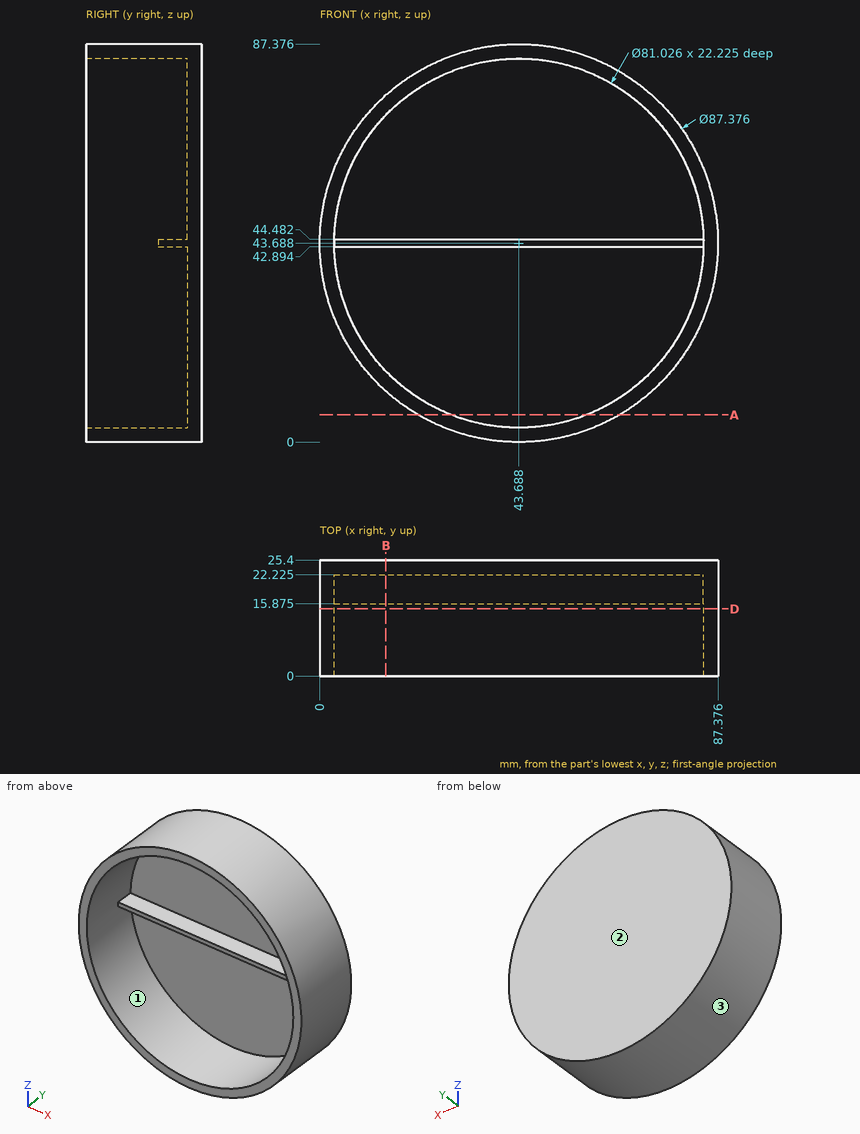
Answer from the drawing. Dimensions are ordinates in mm from the lowest x, y and z of the part. Coordinates: 2 decimals unless noted, no trailing zeros. Order: outer loops, then holes, each group sorted by start corner. A loop starts at its lowest first (then second) coordinate and runs counter-clockwise, first axis right, second up. Notation, with made-up numbers: (-38.5, 83) - (17.5, 83) arc R30 cw to (17.5, 117) - close; hole circle Ø9 at (38.25, 21). An arc over 180 degrees is marked (long way). Answer as a JSON object with one key per item and string values. Group by question number.
Item 1: Consider probe 1 along Z at (x, y) = (43.5, 4.5) (1 decimal); probe 2 along Y at (x, z) = (31.5, 46.5) (1 decimal); probe 3 along X at (y, z) = (18.25, 16) (1 decimal). Determine where each line is inside the solid, lowest interval first. Write a range as from..to.
Item 2: Section A-A (z = 6) is taken. Give the vertices of the cut face in (x, y) (1 decimal).
Item 3: Section B-B (x = 14.5) is taken. Give the vertices of the cut face in (y, z) (1 decimal).
Item 4: Flat-ended cylindrical pins translate along their axes: P1, Ø1.5, axis at y = 11, z = 43.5, coming from the -X side; P2, Ø0.8, axis at x = 30, z = 44, coming from the -Y side (3 decimals); P3, Ø1.9, axis at x = 32, y = 19.5, coming from the +Z side. Find the tip coordinate at first contact, or state that the pin passes through.
Item 5: The mould has two halves that part along Z. Classify the marked faces 1, 2 and 3: +Z half, -Z half, draft (parallel to the pull), parting line (faces both ways), or undercut.
Item 6: Section D-D (y = 14.75) is taken. Give the vertices of the cut face in (x, z) (1 decimal).
Results are:
{
 "1": {"probe 1": "z = 0..3.2, 84.2..87.4", "probe 2": "y = 22.2..25.4", "probe 3": "x = 9.9..14.1, 73.3..77.5"},
 "2": {"outline": "(21.6, 0) - (28.8, 0) - (28.8, 22.2) - (58.6, 22.2) - (58.6, 0) - (65.8, 0) - (65.8, 25.4) - (21.6, 25.4) - close"},
 "3": {"outline": "(0, 11.2) - (25.4, 11.2) - (25.4, 76.2) - (0, 76.2) - (0, 71.8) - (22.2, 71.8) - (22.2, 44.5) - (15.9, 44.5) - (15.9, 42.9) - (22.2, 42.9) - (22.2, 15.6) - (0, 15.6) - close"},
 "4": {"P1": "stops at x = 0", "P2": "stops at y = 15.875", "P3": "stops at z = 86.04"},
 "5": {"face 1": "undercut", "face 2": "draft", "face 3": "parting line"},
 "6": {"outline": "circle Ø87.4 at (43.7, 43.7); hole circle Ø81 at (43.7, 43.7)"}
}
